Autodesk Fusion 360 part; units mm, degrees
sketch "Sketch2" plane through (0, 0, 0) normal (0, 0, 1) x (1, 0, 0)
  line L0 (152.5, -152.5) -> (-152.5, -152.5)
  line L1 (-152.5, -152.5) -> (-152.5, 152.5)
  line L2 (-152.5, 152.5) -> (152.5, 152.5)
  line L3 (152.5, 152.5) -> (152.5, -152.5)
  line L4 (120, -120) -> (-120, -120)
  line L5 (-120, -120) -> (-120, 120)
  line L6 (-120, 120) -> (120, 120)
  line L7 (120, 120) -> (120, -120)
  line L8 (120, -120) -> (-120, 120) construction
  line L9 (-120, -120) -> (120, 120) construction
  circle A0 centre (120, 120) radius 6
  circle A1 centre (-120, 120) radius 6
  circle A2 centre (-120, -120) radius 6
  circle A3 centre (120, -120) radius 6
  circle A4 centre (0, 0) radius 6
  dimension "d6" = 305
  dimension "d7" = 305
  dimension "d8" = 240
  dimension "d9" = 240
  dimension "d10" = 12
  dimension "d12" = 360
  dimension "d15" = 12
extrude "Extrude1" add sketch "Sketch2" along normal blind 1 contours L0 L1 L2 L3 | L4 L5 L6 L7 A0 A1 A2 A3
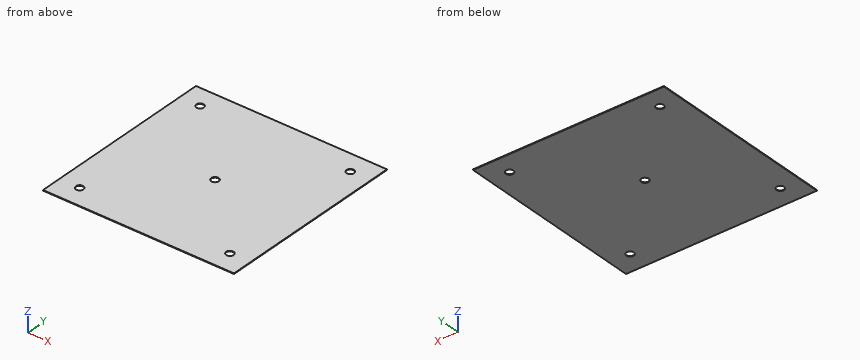
Work out the finished part from the listing and answer in its coordinate system (mm). Give positions to 0.01 mm unless a question says otherwise; leave off trailing zeros. Write each loop counter-clockwise with the first axis right and the second up, starting at its lowest first coordinate (ties: lowest second). Pieces come first, ordered by that corner, then holes. Notation, with made-up numbers: (55.25, -39.5) - (87.25, -39.5) arc R27 cw to (87.25, -6.5) - close; hole circle Ø2 at (-1, 73). An arc over 180 degrees is marked (long way). One line per item, written item: value. Start each with the question number.
1. Find section C-C (x = 0). Write down the section's boundary in (y, z), then the cut area to 3 significant figures.
2. Find section A-A (x = -120). Write down the section's boundary in (y, z), then the cut area to 3 significant figures.
3. Consider probe 1 along X at (y, z) = (-120, 0.4); probe 2 along X at (y, z) = (115, 0.35). Determine where each line is inside the solid, lowest interval first.
Geometry results:
1. outline: (-152.5, 0) - (-6, 0) - (-6, 1) - (-152.5, 1) - close; (6, 0) - (152.5, 0) - (152.5, 1) - (6, 1) - close
1. area: 293 mm2
2. outline: (-152.5, 0) - (-126, 0) - (-126, 1) - (-152.5, 1) - close; (-114, 0) - (114, 0) - (114, 1) - (-114, 1) - close; (126, 0) - (152.5, 0) - (152.5, 1) - (126, 1) - close
2. area: 281 mm2
3. probe 1: -152.5 to -126, -114 to 114, 126 to 152.5
3. probe 2: -152.5 to -123.32, -116.68 to 116.68, 123.32 to 152.5
